from build123d import *

# Parameters (mm, degrees)
F1_DEPTH = 63.5
F2_DEPTH = 25.4
F3_DEPTH = 7.9375
F5_R     = 6.35


# Not quite as in the source:
# - the program builds the solid bodies; features that only make, move or delete a surface that nothing else refers to are left out


with BuildPart() as f1:
    # F0 (on Front) → F1 (new body, symmetric)
    with BuildSketch(Plane.XZ):
        Polygon((22.225, 9.525), (-41.275, 9.525), (-41.275, -9.525), (41.275, -9.525), (41.275, 9.525), align=None)
    extrude(amount=F1_DEPTH, both=True)

    # F0 (on Front) → F2 (join, symmetric)
    with BuildSketch(Plane.XZ):
        with BuildLine():
            Line((22.225, 46.0502), (22.225, 9.525))
            Line((22.225, 9.525), (41.275, 9.525))
            Line((41.275, 9.525), (41.275, 46.0502))
            ThreePointArc((41.275, 46.0502), (45.9246798487, 57.2755201513), (57.15, 61.9252))
            Line((57.15, 61.9252), (60.325, 61.9252))
            Line((60.325, 61.9252), (60.325, 80.9752))
            Line((60.325, 80.9752), (57.15, 80.9752))
            ThreePointArc((57.15, 80.9752), (32.4542956671, 70.7459043329), (22.225, 46.0502))
        make_face()
    extrude(amount=F2_DEPTH, both=True)

    # F0 (on Front) → F3 (join, symmetric)
    with BuildSketch(Plane.XZ):
        with BuildLine():
            add(Edge.make_bspline(
                [(-41.275, 9.525), (-28.4558665007, 41.9093370438), (15.8414896578, 82.5819298625), (57.15, 80.9752)],
                knots=[0, 0, 0, 0, 121.6248811101, 121.6248811101, 121.6248811101, 121.6248811101], degree=3))
            Line((-41.275, 9.525), (22.225, 9.525))
            Line((22.225, 9.525), (22.225, 46.0502))
            ThreePointArc((22.225, 46.0502), (32.4542956671, 70.7459043329), (57.15, 80.9752))
        make_face()
    extrude(amount=F3_DEPTH, both=True)

    # F5
    f5_edges = [f1.edges().sort_by_distance(p)[0] for p in [
        (-41.275, -63.5, 0),
        (41.275, -63.5, 0),
        (41.275, 63.5, 0),
        (-41.275, 63.5, 0),
    ]]
    fillet(f5_edges, radius=F5_R)


solid = f1.part
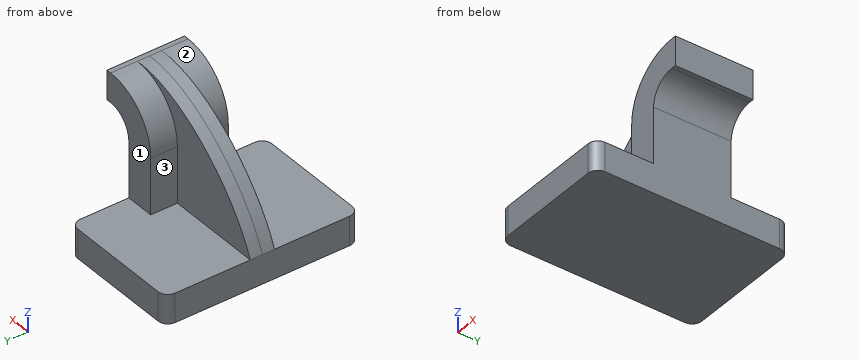
Can you work these out from the model? Positions are in its coordinate system, mm. Face numbers are marked on the shaded views. A direction names the side the tool comes from. Coordinates: 2 decimals unless noted, no trailing zeros. Write each loop counter-clockwise with the first axis right and the second up, starting at its lowest first coordinate (ties: lowest second). Pieces come first, ordered by that corner, then holes. Notation, with made-up numbers: (-19.75, 83) -> (1.25, 83) arc R28 cw to (1.25, 104) -> close; hole circle Ø1 at (0.5, 79.25). An arc over 180 degrees is marked (long way). Answer as CSV lines item,"result".
1) If I drill on line 1 (X direction, y = -9, z = 16.5) (3 decimals); line 2 (Z direction, x = 2.5, y = -9.5) (3 decimals); line 3 (Y direction, x = -34.5, z = 17.5), over which ranges is the centre line in solid material (lowest first)? Write a range as from..to.
Check result:
line 1,"22.225..41.275"
line 2,"-9.525..9.525"
line 3,"-7.94..7.94"
2) If we section it at B-B on y = -21: Please give me the cut outline in (x, z) (3 decimals).
Check result:
outline,"(-41.275, -9.525) -> (41.275, -9.525) -> (41.275, 46.05) arc R15.875 cw to (57.15, 61.925) -> (60.325, 61.925) -> (60.325, 80.975) -> (57.15, 80.975) arc R34.925 ccw to (22.225, 46.05) -> (22.225, 9.525) -> (-41.275, 9.525) -> close"
3) If we section it at C-C on y = -47: Please give me the cut outline in (x, z) (3 decimals).
Check result:
outline,"(-41.275, -9.525) -> (41.275, -9.525) -> (41.275, 9.525) -> (-41.275, 9.525) -> close"
4) Will these pins go through, and if not, where does the flat tip stop? P1, Ø21.5, axis at x = 2, z = 34, coming from the +Y side; P2, Ø3.5, axis at x = 58, y = -10, coming from the -Z side; P3, Ø2, axis at x = 2, y = 27, coming from the +Z side (3 decimals).
Check result:
P1,"y = 7.94"
P2,"z = 61.9"
P3,"z = 9.525"
5) On a 3-axis mill with a long thin cutter (end or side, diameter ignored), from which of +Z, -Z, +X, -X, +Y, -Y can I reach the whole of each face in a straight line? I mean the marked faces 1, 2 and 3. Say none if no direction works.
Check result:
face 1,"+Z, +X, -X, +Y"
face 2,"+Z, -X, -Y"
face 3,"+Z, -X, +Y"
6) If we section it at A-A on z = -1.5: Please give me the cut outline in (x, y) (3 decimals), then the cut area to 3 significant figures.
Check result:
outline,"(-41.275, -57.15) arc R6.35 ccw to (-34.925, -63.5) -> (34.925, -63.5) arc R6.35 ccw to (41.275, -57.15) -> (41.275, 57.15) arc R6.35 ccw to (34.925, 63.5) -> (-34.925, 63.5) arc R6.35 ccw to (-41.275, 57.15) -> close"
area,"10,400 mm²"
